Work out the finished part from the listing and answer in its coordinate system (mm). A direction names the side the tool comes from. Round coordinates to 2 decimals unless told otherwise and drop trailing zeros. Loops run counter-clockwise (first coordinate to the right, second up) from the corner with the lowest first, then second, coordinate; pieces in that order, holes last. Notation, with made-up numbers: (70.5, 2) - (99.5, 2) arc R16 cw to (99.5, 8) - close; hole circle Ø10 at (18.5, -23.75). An arc over 180 degrees is marked (long way). Return JSON: item names as keys, results as strings.
from build123d import *

# Parameters (mm, degrees)
SKETCH7_R                         = 158.75
SKETCH7_R_2                       = 152.4
SKETCH7_R_3                       = 127
BOSS_EXTRUDE2_DEPTH               = 6.35
SKETCH7_3_R                       = 127
SKETCH7_3_R_2                     = 114.3
BOSS_EXTRUDE3_DEPTH               = 31.75
PIPE_TAP_DRILL_FOR_1_2_TAP2_D     = 17.8562
PIPE_TAP_DRILL_FOR_1_2_TAP2_DEPTH = 31.75
PIPE_TAP_DRILL_FOR_1_2_TAP2_TIP   = 5.364543693
F_1_2_0_5_DIAMETER_HOLE3_D        = 12.7
F_1_2_0_5_DIAMETER_HOLE3_DEPTH    = 62.23
F_1_2_0_5_DIAMETER_HOLE3_TIP      = 3.815464931
F_1_2_0_5_DIAMETER_HOLE4_D        = 12.7
F_1_2_0_5_DIAMETER_HOLE4_DEPTH    = 39.37
F_1_2_0_5_DIAMETER_HOLE4_TIP      = 3.815464931
F_10_CLEARANCE_HOLE1_D            = 4.9784
CIRPATTERN1_COUNT                 = 8


with BuildPart() as part:
    # Sketch7 → Boss-Extrude2 (new body)
    with BuildSketch(Plane(origin=(0, 0, 0), x_dir=(1, 0, 0), z_dir=(0, 1, 0))):
        Circle(SKETCH7_R)
        Circle(SKETCH7_R_2, mode=Mode.SUBTRACT)
        Circle(SKETCH7_R_2)
        Circle(SKETCH7_R_3, mode=Mode.SUBTRACT)
    extrude(amount=-BOSS_EXTRUDE2_DEPTH)

    # Sketch7_3 → Boss-Extrude3 (add)
    with BuildSketch(Plane(origin=(0, 0, 0), x_dir=(1, 0, 0), z_dir=(0, 1, 0))):
        Circle(SKETCH7_3_R)
        Circle(SKETCH7_3_R_2, mode=Mode.SUBTRACT)
        with BuildLine():
            Line((-100.803124952, -25.4), (-111.44204772, -25.4))
            ThreePointArc((-111.44204772, -25.4), (-100.637932046, -54.189451312), (-82.55, -79.056862447))
            Line((-82.55, -79.056862447), (-82.55, -73.780332745))
            Line((-82.55, -73.780332745), (-82.55, -25.4))
            Line((-82.55, -25.4), (-100.803124952, -25.4))
        make_face()
        with BuildLine():
            ThreePointArc((-113.403515571, -14.2875), (-112.560000653, -19.867970533), (-111.44204772, -25.4))
            Line((-111.44204772, -25.4), (-100.803124952, -25.4))
            ThreePointArc((-100.803124952, -25.4), (-109.203385364, -22.225), (-113.403515571, -14.2875))
        make_face()
        with BuildLine():
            Line((-82.55, -73.780332745), (-82.55, -79.056862447))
            ThreePointArc((-82.55, -79.056862447), (-80.589780271, -81.054162854), (-78.58125, -83.002874338))
            ThreePointArc((-78.58125, -83.002874338), (-81.5156949, -78.800448531), (-82.55, -73.780332745))
        make_face()
    extrude(amount=-BOSS_EXTRUDE3_DEPTH)

    # Pipe Tap Drill for 1_2 Tap2
    with Locations(Plane(origin=(0, -12.7, 12.7), x_dir=(1, 0, 0), z_dir=(0, 0.707106781, -0.707106781))):
        with Locations((-95.25, -30.660512242)):
            Hole(PIPE_TAP_DRILL_FOR_1_2_TAP2_D / 2, depth=PIPE_TAP_DRILL_FOR_1_2_TAP2_DEPTH)
            with Locations((0, 0, -(PIPE_TAP_DRILL_FOR_1_2_TAP2_DEPTH + PIPE_TAP_DRILL_FOR_1_2_TAP2_TIP / 2))):  # 118° drill point
                Cone(0, PIPE_TAP_DRILL_FOR_1_2_TAP2_D / 2, PIPE_TAP_DRILL_FOR_1_2_TAP2_TIP, mode=Mode.SUBTRACT)

    # 1_2 _0.5_ Diameter Hole3
    with Locations(Plane.XY.offset(127)):
        with Locations((-95.25, -19.05)):
            Hole(F_1_2_0_5_DIAMETER_HOLE3_D / 2, depth=F_1_2_0_5_DIAMETER_HOLE3_DEPTH)
            with Locations((0, 0, -(F_1_2_0_5_DIAMETER_HOLE3_DEPTH + F_1_2_0_5_DIAMETER_HOLE3_TIP / 2))):  # 118° drill point
                Cone(0, F_1_2_0_5_DIAMETER_HOLE3_D / 2, F_1_2_0_5_DIAMETER_HOLE3_TIP, mode=Mode.SUBTRACT)

    # 1_2 _0.5_ Diameter Hole4
    with Locations(Plane(origin=(0, -12.7, 12.7), x_dir=(1, 0, 0), z_dir=(0, 0.707106781, -0.707106781))):
        with Locations((-95.25, -30.660512242)):
            Hole(F_1_2_0_5_DIAMETER_HOLE4_D / 2, depth=F_1_2_0_5_DIAMETER_HOLE4_DEPTH)
            with Locations((0, 0, -(F_1_2_0_5_DIAMETER_HOLE4_DEPTH + F_1_2_0_5_DIAMETER_HOLE4_TIP / 2))):  # 118° drill point
                Cone(0, F_1_2_0_5_DIAMETER_HOLE4_D / 2, F_1_2_0_5_DIAMETER_HOLE4_TIP, mode=Mode.SUBTRACT)

    # 10 Clearance Hole1 (through all)
    with Locations(Plane(origin=(0, 0, 0), x_dir=(1, 0, 0), z_dir=(0, 1, 0))):
        with Locations((0, -120.65)):
            f_10_clearance_hole1 = Hole(F_10_CLEARANCE_HOLE1_D / 2)

    # CirPattern1: 10 Clearance Hole1 ×8 about axis
    cirpattern1_axis = Axis((0, 0, 0), (0, 1, 0))
    for i in range(1, CIRPATTERN1_COUNT):
        add(f_10_clearance_hole1.rotate(cirpattern1_axis, i * 360 / CIRPATTERN1_COUNT), mode=Mode.SUBTRACT)


solid = part.part
1) Find the intervals of material crossed by L1, parallel to X at y = -23.5, z = 0; L2, parallel to X at y = -6, z = 0; L3, parallel to X at y = -19.05, z = 70.75, in increasing order.
Verdict:
{"L1": "x = -127 to -123.14, -118.16 to -114.3, 114.3 to 118.16, 123.14 to 127", "L2": "x = -158.75 to -123.14, -118.16 to -114.3, 114.3 to 118.16, 123.14 to 158.75", "L3": "x = -105.47 to -101.6, -88.9 to -82.55, 89.77 to 105.47"}
2) Determine the mould class of faces 1 (the flat face through (-82.55, -16, 50)), 2 (the cylindrical face through (-94.42, -21.19, 55.65)), 3 (the flat face through (-108, 0, 33)), 4 (the flat face through (-71, -6.35, -107)) for opening direction Y: pulls with the +Y half, pulls with the -Y half, needs draft (parallel to the pull), parting line crosses it, or undercut.
Verdict:
{"face 1": "needs draft", "face 2": "undercut", "face 3": "pulls with the +Y half", "face 4": "pulls with the -Y half"}
3) A tool of negligible diameter and unlimited length cuts with its end or side. For faces 5 (the cylindrical face through (121.135, -18.872, -38.147)), 6 (the cylindrical face through (-88.906, -18.771, 74.671)), 7 (the cylindrical face through (-81.487, -15.653, 78.867)), from which of +Z, -Z, +X, -X, +Y, -Y can it reach the whole face along a straight path? Write none if from no direction.
Verdict:
{"face 5": "-Y", "face 6": "+Z", "face 7": "+Y, -Y"}
4) Section B-B (x = 36.5) is taken. Give the vertices of the cut face in (y, z).
Verdict:
{"outline": "(-31.75, -121.64) - (-6.35, -121.64) - (-6.35, -154.5) - (0, -154.5) - (0, -108.32) - (-31.75, -108.32) - close; (-31.75, 108.32) - (0, 108.32) - (0, 154.5) - (-6.35, 154.5) - (-6.35, 121.64) - (-31.75, 121.64) - close"}
5) Section A-A (x = -39) is taken. Give the vertices of the cut face in (y, z), and give its area (3 significant figures).
Verdict:
{"outline": "(-31.75, -120.86) - (-6.35, -120.86) - (-6.35, -153.88) - (0, -153.88) - (0, -107.44) - (-31.75, -107.44) - close; (-31.75, 107.44) - (0, 107.44) - (0, 153.88) - (-6.35, 153.88) - (-6.35, 120.86) - (-31.75, 120.86) - close", "area": "1,270 mm2"}
6) Flat-ended cylindrical pins translate along their axes: pin 1 (12 mm diameter, centred on x = 71, y = -16.5, fed in from +Z); pin 2 (3 mm diameter, centred on x = 0, z = 120.65, fed in from +Y); pin 3 (10 mm diameter, centred on y = -16, z = 41, fed in from -X); pin 4 (2 mm diameter, centred on x = 25, y = -3.5, fed in from +Z). Find the tip coordinate at first contact, or state that the pin passes through.
Verdict:
{"pin 1": "stops at z = 109.11", "pin 2": "passes through", "pin 3": "stops at x = -121.79", "pin 4": "stops at z = 156.93"}
